Part model, mm, in its own coordinate system. Round coordinates to 2 decimals unless told otherwise and drop trailing zeros. Write each loop counter-clockwise with the first axis right and the second up, starting at its lowest first coordinate (ties: lowest second). Pieces come first, ordered by that corner, then holes. Notation, with made-up numbers: M 44.5,66 L 69.5,66 A14 ccw 69.5,79 Z; hole C 51,-12.5 d1. An arc over 180 degrees is marked long. Use one line per item in the form item = value. Start each with the question number.
Item 1: Cut at B-B, the plane y = -120. Give the cut face in (x, z).
Item 2: Cut at A-A, the plane z = 0.2. State how many separate pieces and enclosed holes the cut face has, then the cut area to 3 significant figures.
Item 3: Probe L1, parallel to X at y = -60.5, z = 0.2; L2, parallel to Y at x = -144.5, z = 0.65; L3, parallel to Y at x = -115, z = 0.7. List the from-to ranges inside material, lowest first.
Item 4: Mould opens along X. For faces 1 (the face through (-133.458, -155.487, 0.493)), 2 (the face through (-3, 4, 1)) say: +X half, -X half, draft (parallel to the pull), parting line (faces both ways), or undercut.
from build123d import *

# Parameters (mm, degrees)
SKETCH_1_W          = 470
SKETCH_1_H          = 600
EXTRUDE_1_DEPTH     = 1
HOLE_WIZARD_M5_1_D  = 5.5
SKETCH_4_R          = 40
CUT_EXTRUDE_1_DEPTH = 10


with BuildPart() as part:
    # 스케치1 → 보스-돌출1 (new body)
    with BuildSketch(Plane.XY):
        Rectangle(SKETCH_1_W, SKETCH_1_H)
    extrude(amount=EXTRUDE_1_DEPTH)

    # M5 여유 구멍1 (through all)
    with Locations(Plane(origin=(0, 0, 0), x_dir=(-1, 0, 0), z_dir=(0, 0, -1))):
        with Locations((-225, 290), (-135, 290), (-45, 290), (45, 290), (135, 290), (225, 290), (225, 174), (225, 58), (225, -58), (225, -174), (225, -290), (-225, 174), (-225, 58), (-225, -58), (-225, -174), (-225, -290), (-135, -290), (-45, -290), (45, -290), (135, -290)):
            Hole(HOLE_WIZARD_M5_1_D / 2)

    # 스케치4 → 컷-돌출1 (cut)
    with BuildSketch(Plane(origin=(0, 0, 0), x_dir=(-1, 0, 0), z_dir=(0, 0, -1))):
        with Locations((115, -120)):
            Circle(SKETCH_4_R)
    extrude(amount=-CUT_EXTRUDE_1_DEPTH, mode=Mode.SUBTRACT)


solid = part.part
Model answer:
q1.outline = M -235,0 L -155,0 L -155,1 L -235,1 Z; M -75,0 L 235,0 L 235,1 L -75,1 Z
q2.separate_pieces = 1
q2.enclosed_holes = 21
q2.area = 276,000 mm²
q3.L1 = -235 to -226.15, -223.85 to 223.85, 226.15 to 235
q3.L2 = -300 to -147.01, -92.99 to 300
q3.L3 = -300 to -160, -80 to 300
q4.face_1 = undercut
q4.face_2 = draft
